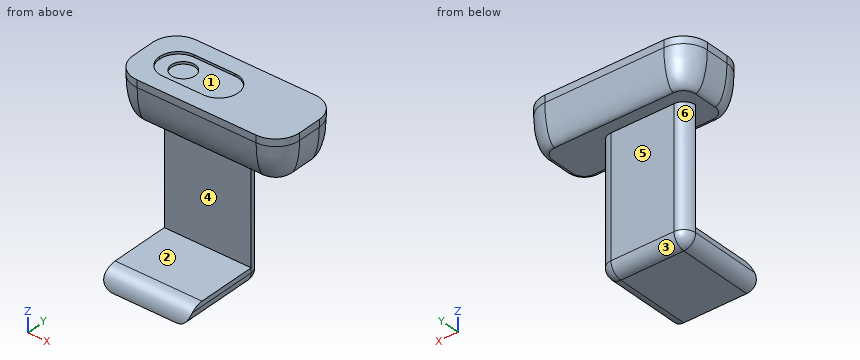
from build123d import *

# Parameters (mm, degrees)
RESSALTO_EXTRUS_O1_DEPTH = 18
FILETE1_SIZE             = 15
FILETE1_SIZE_2           = 5
ESBO_O2_R                = 5
CORTE_EXTRUS_O1_DEPTH    = 2
CORTE_EXTRUS_O2_DEPTH    = 1
ESBO_O4_W                = 36.5
ESBO_O4_H                = 5
RESSALTO_EXTRUS_O2_DEPTH = 55
FILETE2_R                = 5
ESBO_O5_W                = 36.5
ESBO_O5_H                = 7
RESSALTO_EXTRUS_O3_DEPTH = 32
FILETE3_R                = 5
FILETE4_R                = 7


# Some blends are built 0.0001 mm under size
with BuildPart() as part:
    # Esboço1 → Ressalto-extrusão1 (new body)
    with BuildSketch(Plane.XY):
        with BuildLine():
            Line((-25, -15), (25, -15))
            ThreePointArc((25, -15), (32.071067812, -12.071067812), (35, -5))
            Line((35, -5), (35, 5))
            ThreePointArc((35, 5), (32.071067812, 12.071067812), (25, 15))
            Line((25, 15), (-25, 15))
            ThreePointArc((-25, 15), (-32.071067812, 12.071067812), (-35, 5))
            Line((-35, 5), (-35, -5))
            ThreePointArc((-35, -5), (-32.071067812, -12.071067812), (-25, -15))
        make_face()
    extrude(amount=RESSALTO_EXTRUS_O1_DEPTH)

    # Filete1
    # an asymmetric fillet: 15, 5 mm, written as the material it takes off along each edge
    with BuildSketch(Plane(origin=(25, 15, 0), x_dir=(0, 0, 1), z_dir=(-1, 0, 0)), Plane(origin=(-25, -15, 0), x_dir=(0, 0, 1), z_dir=(1, 0, 0))) as filete1_piece_1:
        with BuildLine():
            Bezier((FILETE1_SIZE, 0), (0, 0), (0, -FILETE1_SIZE_2), weights=[1, 0.707106781, 1])
            Line((0, -FILETE1_SIZE_2), (0, 0))
            Line((0, 0), (FILETE1_SIZE, 0))
        make_face()
    extrude(amount=50, mode=Mode.SUBTRACT)
    with BuildSketch(Plane(origin=(25, 5, 0), x_dir=(1, 0, 0), z_dir=(0, -1, 0))) as filete1_piece_2:
        with BuildLine():
            Bezier((10, FILETE1_SIZE), (10, 0), (10 - FILETE1_SIZE_2, 0), weights=[1, 0.707106781, 1])
            Line((10 - FILETE1_SIZE_2, 0), (10, 0))
            Line((10, 0), (10, FILETE1_SIZE))
        make_face()
    revolve(axis=Axis((25, 5, 0), (0, 0, 1)), revolution_arc=90, mode=Mode.SUBTRACT)
    with BuildSketch(Plane(origin=(35, -5, 0), x_dir=(0, 0, 1), z_dir=(0, 1, 0)), Plane(origin=(-35, 5, 0), x_dir=(0, 0, 1), z_dir=(0, -1, 0))) as filete1_piece_3:
        with BuildLine():
            Bezier((FILETE1_SIZE, 0), (0, 0), (0, -FILETE1_SIZE_2), weights=[1, 0.707106781, 1])
            Line((0, -FILETE1_SIZE_2), (0, 0))
            Line((0, 0), (FILETE1_SIZE, 0))
        make_face()
    extrude(amount=10, mode=Mode.SUBTRACT)
    with BuildSketch(Plane(origin=(25, -5, 0), x_dir=(0, -1, 0), z_dir=(-1, 0, 0))) as filete1_piece_4:
        with BuildLine():
            Bezier((10, FILETE1_SIZE), (10, 0), (10 - FILETE1_SIZE_2, 0), weights=[1, 0.707106781, 1])
            Line((10 - FILETE1_SIZE_2, 0), (10, 0))
            Line((10, 0), (10, FILETE1_SIZE))
        make_face()
    revolve(axis=Axis((25, -5, 0), (0, 0, 1)), revolution_arc=90, mode=Mode.SUBTRACT)
    with BuildSketch(Plane(origin=(-25, -5, 0), x_dir=(-1, 0, 0), z_dir=(0, 1, 0))) as filete1_piece_5:
        with BuildLine():
            Bezier((10, FILETE1_SIZE), (10, 0), (10 - FILETE1_SIZE_2, 0), weights=[1, 0.707106781, 1])
            Line((10 - FILETE1_SIZE_2, 0), (10, 0))
            Line((10, 0), (10, FILETE1_SIZE))
        make_face()
    revolve(axis=Axis((-25, -5, 0), (0, 0, 1)), revolution_arc=90, mode=Mode.SUBTRACT)
    with BuildSketch(Plane(origin=(-25, 5, 0), x_dir=(0, 1, 0), z_dir=(1, 0, 0))) as filete1_piece_6:
        with BuildLine():
            Bezier((10, FILETE1_SIZE), (10, 0), (10 - FILETE1_SIZE_2, 0), weights=[1, 0.707106781, 1])
            Line((10 - FILETE1_SIZE_2, 0), (10, 0))
            Line((10, 0), (10, FILETE1_SIZE))
        make_face()
    revolve(axis=Axis((-25, 5, 0), (0, 0, 1)), revolution_arc=90, mode=Mode.SUBTRACT)

    # Esboço2 → Corte-extrusão1 (cut)
    with BuildSketch(Plane.XY.offset(18)):
        with Locations((-18, 0)):
            Circle(ESBO_O2_R)
    extrude(amount=-CORTE_EXTRUS_O1_DEPTH, mode=Mode.SUBTRACT)

    # Esboço3 → Corte-extrusão2 (cut)
    with BuildSketch(Plane.XY.offset(18)):
        with BuildLine():
            Line((-2.9, -8), (-20.1, -8))
            ThreePointArc((-20.1, -8), (-25.686143571, -5.686143571), (-28, -0.1))
            Line((-28, -0.1), (-28, 0.1))
            ThreePointArc((-28, 0.1), (-25.686143571, 5.686143571), (-20.1, 8))
            Line((-20.1, 8), (-2.9, 8))
            ThreePointArc((-2.9, 8), (2.686143571, 5.686143571), (5, 0.1))
            Line((5, 0.1), (5, -0.1))
            ThreePointArc((5, -0.1), (2.686143571, -5.686143571), (-2.9, -8))
        make_face()
    extrude(amount=-CORTE_EXTRUS_O2_DEPTH, mode=Mode.SUBTRACT)

    # Esboço4 → Ressalto-extrusão2 (add)
    with BuildSketch(Plane(origin=(0, 0, 0), x_dir=(-1, 0, 0), z_dir=(0, 0, -1))):
        with Locations((7.75, 2.5)):
            Rectangle(ESBO_O4_W, ESBO_O4_H)
    extrude(amount=RESSALTO_EXTRUS_O2_DEPTH)

    # Filete2
    filete2_edges = [part.edges().sort_by_distance(p)[0] for p in [
        (-26, 5, -27.5),
        (10.5, 5, -27.5),
    ]]
    fillet(filete2_edges, radius=FILETE2_R - 0.0001)  # a hair under: the kernel refuses the full size

    # Esboço5 → Ressalto-extrusão3 (add)
    with BuildSketch(Plane.XZ):
        with Locations((-7.75, -51.5)):
            Rectangle(ESBO_O5_W, ESBO_O5_H)
    extrude(amount=RESSALTO_EXTRUS_O3_DEPTH)

    # Filete3
    filete3_edges = [part.edges().sort_by_distance(p)[0] for p in [
        (-7.75, 5, -55),
        (9.035563195, 3.535563195, -55),
        (-24.535563195, 3.535563195, -55),
        (-26, -15.99995, -55),
        (10.5, -15.99995, -55),
    ]]
    fillet(filete3_edges, radius=FILETE3_R - 0.0001)  # a hair under: the kernel refuses the full size

    # Filete4
    filete4_edges = [part.edges().sort_by_distance(p)[0] for p in [
        (-7.75, -32, -48),
    ]]
    fillet(filete4_edges, radius=FILETE4_R - 0.0001)  # a hair under: the kernel refuses the full size


solid = part.part
Source: CAD feature listing. Evaluate the final solid. Frame: model axes, mm. Face numbers are marked on the shaded views. A direction names the side the tool comes from. Give positions to 0.01 mm unless a question says otherwise; leave off trailing zeros. Use a Markdown table: item, result. Add a question column.
1) Reachability of the marked faces 4, 5 and 6 from +Z, -Z, +X, -X, +Y, -Y: full face, straight path, thin tool, end or side. Return the list, or none.
2) Pull-direction query (Y, two-part tool) for the marked faces 1, 2 and 3; classes: +Y half, -Y half, draft (parallel to the pull), parting line (faces both ways), or undercut.
3) First-contact query: pin 1 (8 mm diameter, centred on x = 3, y = -4, fed in from +Z); pin 2 (11 mm diameter, centred on x = -12.5, z = -20.5, fed in from -Y); pin 3 (0.5 mm diameter, centred on x = -8.5, z = 17.5, fed in from -Y); pin 4 (2 mm diameter, centred on x = -14.5, z = 1, fed in from -Y). Flat tips, straight axial feed; report the tip coordinate or a pass-through.
4) Line query: line 1 along Y through (x, z) = (-18, 16.75); line 2 along Y through (x, z) = (-18, -39); line 3 along Z through (x, y) = (20, -6.5). Output: solid intervals per line, ascending. Write a range as [from, to].
Numbers:
| question | item | result |
|---|---|---|
| 1 | face 4 | +X, -X, -Y |
| 1 | face 5 | -Z, +X, -X, +Y |
| 1 | face 6 | -Z, -X, +Y |
| 2 | face 1 | undercut |
| 2 | face 2 | draft |
| 2 | face 3 | +Y half |
| 3 | pin 1 | stops at z = 18 |
| 3 | pin 2 | stops at y = 0 |
| 3 | pin 3 | stops at y = -15 |
| 3 | pin 4 | stops at y = -12.49 |
| 4 | line 1 | y = [-15, -5], [5, 15] |
| 4 | line 2 | y = [0, 5] |
| 4 | line 3 | z = [0, 18] |
